Geometry: final body of the model. Coordinates: model frame, mm. A direction names the side the tool comes from. Give positions to 0.01 mm unless a question says otherwise; leave off trailing zeros. Order: outer loops, then holes, each group sorted by start corner. A loop starts at its lowest first (then second) coordinate and runs counter-clockwise, first axis right, second up. Notation, with made-up numbers: (18.25, -14) -> (76.25, -14) arc R14 cw to (76.25, 6) -> close; hole circle Ø10 at (13, 31.25). An arc over 180 degrees is marked (long way). One line per question, with ' | ' between items. Start each with the question number.
(1) Section C-C (x = 18). Return loops of the section in (y, z).
(2) Mould query, pull axis Z, two halves, no side actions, for faces 5 (the face through (0, 3, -35)), 6 (the face through (10, 9, 26)), 7 (the face through (9, 17, 11)). Classes: +Z half, -Z half, draft (parallel to the pull), parting line (faces both ways), or undercut.
(3) Ray query, L1, parallel to X at y = 7.25, z = 34.5; L2, parallel to X at y = 11.25, z = -12; L3, parallel to Y at x = -3.5, z = -13. Return the intervals inside material, ascending.
(4) Section D-D (z = 0.5). Return loops of the section in (x, y), then the cut area to 3 significant figures.
(5) Section A-A (y = 5.25). Return loops of the section in (x, z), then the cut area to 3 significant figures.
(6) Set-up query: faces 1 (the face through (-21.895, 11.93, 7.284)), 2 (the face through (-9.2, 9, 34)), 3 (the face through (-4, 12, 34)), 4 (the face through (-19, 9, 26)). Return all of +Z, -Z, +X, -X, +Y, -Y with unobstructed straight access to the full face (end or side cutting, diameter ignored); none if empty.
(7) First-contact query: pin 1 Ø1.5 at (x, y) = (-16.5, 10.5) entering from -Z; pin 2 Ø3.5 at (x, y) = (5.5, 6.5) entering from +Z; pin 3 Ø1.5 at (y, z) = (10, 34.5) entering from +X. Flat tips, straight axial feed; report the tip coordinate or a pass-through.
(8) Section B-B (z = -12). Return loops of the section in (x, y), then the cut area to 3 significant figures.
```python
from build123d import *

# Parameters (mm, degrees)
SKETCH_1_W      = 65
SKETCH_1_H      = 70
EXTRUDE_1_DEPTH = 7
FILLET_1_R      = 2
SKETCH_3_R      = 18
SKETCH_3_R_2    = 9
EXTRUDE_2_DEPTH = 15
SKETCH_4_R      = 4
EXTRUDE_3_DEPTH = 10
SKETCH_5_W      = 10
SKETCH_5_H      = 9
SKETCH_5_H_2    = 8.8
EXTRUDE_4_DEPTH = 5


with BuildPart() as part:
    # 草图1 → 凸台-拉伸1 (new body)
    with BuildSketch(Plane(origin=(0, 0, 0), x_dir=(1, 0, 0), z_dir=(0, 1, 0))):
        Rectangle(SKETCH_1_W, SKETCH_1_H)
    extrude(amount=EXTRUDE_1_DEPTH)

    # 圆角1
    fillet_1_edges = [part.edges().sort_by_distance(p)[0] for p in [
        (32.5, 3.5, 35),
        (-32.5, 3.5, 35),
        (-32.5, 3.5, -35),
        (32.5, 3.5, -35),
    ]]
    fillet(fillet_1_edges, radius=FILLET_1_R)

    # 草图3 → 凸台-拉伸2 (add)
    with BuildSketch(Plane(origin=(0, 7, 0), x_dir=(1, 0, 0), z_dir=(0, 1, 0))):
        with Locations(Location((-9.5, 12, 0), (0, 0, 270))):
            Circle(SKETCH_3_R)
        with Locations(Location((-9.5, 12, 0), (0, 0, 270))):
            Circle(SKETCH_3_R_2, mode=Mode.SUBTRACT)
    extrude(amount=EXTRUDE_2_DEPTH)

    # 草图4 → 凸台-拉伸3 (add)
    with BuildSketch(Plane(origin=(0, 7, 0), x_dir=(1, 0, 0), z_dir=(0, 1, 0))):
        with Locations(Location((-20.693709583, -11.099353322, 0), (0, 0, 90))):
            Circle(SKETCH_4_R)
        with Locations(Location((-10.440917108, -13.544973545, 0), (0, 0, 90))):
            Circle(SKETCH_4_R)
        with Locations(Location((9.12404468, -11.099353322, 0), (0, 0, 90))):
            Circle(SKETCH_4_R)
        with Locations(Location((20.599647266, -20.317460317, 0), (0, 0, 90))):
            Circle(SKETCH_4_R)
        with Locations(Location((-0.846560847, -13.544973545, 0), (0, 0, 90))):
            Circle(SKETCH_4_R)
        with Locations(Location((20.599647266, -11.099353322, 0), (0, 0, 90))):
            Circle(SKETCH_4_R)
    extrude(amount=EXTRUDE_3_DEPTH)

    # 草图5 → 凸台-拉伸4 (add)
    with BuildSketch(Plane(origin=(0, 7, 0), x_dir=(1, 0, 0), z_dir=(0, 1, 0))):
        with Locations((-18.7, -30.5)):
            Rectangle(SKETCH_5_W, SKETCH_5_H)
        with Locations((-4.2, -34.4)):
            Rectangle(SKETCH_5_W, SKETCH_5_H_2)
        with Locations((10.4, -30.5)):
            Rectangle(SKETCH_5_W, SKETCH_5_H)
    extrude(amount=EXTRUDE_4_DEPTH)


solid = part.part
```
Response:
1) outline: (0, -35) -> (7, -35) -> (7, 8.06) -> (17, 8.06) -> (17, 14.14) -> (7, 14.14) -> (7, 17.28) -> (17, 17.28) -> (17, 23.36) -> (7, 23.36) -> (7, 35) -> (0, 35) -> close
2) face 5: -Z half | face 6: undercut | face 7: draft
3) L1: x = -23.7 to -13.7, -9.2 to 0.8, 5.4 to 15.4 | L2: x = -27.5 to -18.5, -0.5 to 8.5 | L3: y = 0 to 7
4) outline: (-32.5, 0) -> (32.5, 0) -> (32.5, 7) -> (3.45, 7) -> (3.45, 22) -> (-22.45, 22) -> (-22.45, 7) -> (-32.5, 7) -> close | area: 844 mm^2
5) outline: (-32.5, -33) arc R2 ccw to (-30.5, -35) -> (30.5, -35) arc R2 ccw to (32.5, -33) -> (32.5, 33) arc R2 ccw to (30.5, 35) -> (-30.5, 35) arc R2 ccw to (-32.5, 33) -> close | area: 4,550 mm^2
6) face 1: +Y | face 2: +Z, +Y | face 3: +Z, +X, -X, +Y | face 4: +X, -X, +Y
7) pin 1: stops at z = -28.88 | pin 2: stops at z = 35 | pin 3: stops at x = 15.4
8) outline: (-32.5, 0) -> (32.5, 0) -> (32.5, 7) -> (8.5, 7) -> (8.5, 22) -> (-0.5, 22) -> (-0.5, 7) -> (-18.5, 7) -> (-18.5, 22) -> (-27.5, 22) -> (-27.5, 7) -> (-32.5, 7) -> close | area: 725 mm^2
